The listing builds one solid part. Answer for the finished solid, in the listing's coordinates (mm). Face numbers are marked on the shaded views. Give positions to 0.01 mm unless a question says otherwise; leave off trailing zeros. Order: outer loops, then holes, each group sorted by start corner. A loop starts at its lowest first (then second) coordinate and runs counter-clockwise, first axis right, second up. Notation, with made-up numbers: (20.5, 62) - (62.5, 62) arc R17 ccw to (62.5, 86) - close; hole circle Ø9 at (53, 87). An arc over 180 degrees is marked (long way). Answer as CSV lines item,"result". Start each with the question number.
1. Section A-A on y = -1.5 is taken. Give the vertices of the cut face in (x, z), and give its area (3 significant figures).
2. Section D-D on x = 0 is taken. Give the vertices of the cut face in (y, z) (1 decimal).
3. Section B-B on x = -2.75 is taken. Give the vertices of the cut face in (y, z).
4. Consider line 1 along X through (y, z) = (2.5, 0.2); line 2 along X through (y, z) = (-2.5, 0); line 3 along X through (y, z) = (-3, 0.1). Determine where each line is inside the solid, lowest interval first. Write a range as [from, to].
5. Determine the mould class of the marked faces 1, 2 and 3 for opening direction Y: +Y half, -Y half, draft (parallel to the pull), parting line (faces both ways), or undercut.
from build123d import *

# Parameters (mm, degrees)
BOSS_EXTRUDE1_DEPTH = 0.3175


with BuildPart() as part:
    # Sketch1 → Boss-Extrude1 (new body, symmetric)
    with BuildSketch(Plane.XY):
        with BuildLine():
            Line((-2.31, 0), (-3.124160712, 0))
            ThreePointArc((-3.124160712, 0), (-2.463203432, 1.921720325), (-0.76, 3.030310241))
            Line((-0.76, 3.030310241), (-0.565, 2.239838164))
            ThreePointArc((-0.565, 2.239838164), (0, 2.31), (0.565, 2.239838164))
            Line((0.565, 2.239838164), (0.76, 3.030310241))
            ThreePointArc((0.76, 3.030310241), (2.463203432, 1.921720325), (3.124160712, 0))
            Line((3.124160712, 0), (2.31, 0))
            ThreePointArc((2.31, 0), (2.103247489, -0.955222487), (1.52, -1.739453937))
            Line((1.52, -1.739453937), (1.80501504, -3.733492135))
            ThreePointArc((1.80501504, -3.733492135), (2.089707078, -4.11637794), (2.565878648, -4.086183031))
            ThreePointArc((2.565878648, -4.086183031), (0, 4.825), (-2.565878648, -4.086183031))
            ThreePointArc((-2.565878648, -4.086183031), (-2.089707078, -4.11637794), (-1.80501504, -3.733492135))
            Line((-1.80501504, -3.733492135), (-1.52, -1.739453937))
            ThreePointArc((-1.52, -1.739453937), (-2.103247489, -0.955222487), (-2.31, 0))
        make_face()
    extrude(amount=BOSS_EXTRUDE1_DEPTH, both=True)


solid = part.part
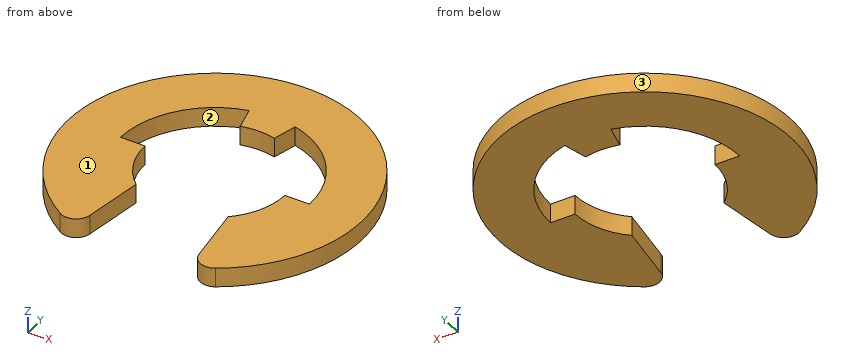
Checks:
1,outline,"(-4.59, -0.32) - (-1.76, -0.32) - (-1.76, 0.32) - (-4.59, 0.32) - close; (1.76, -0.32) - (4.59, -0.32) - (4.59, 0.32) - (1.76, 0.32) - close"
1,area,"3.59 mm²"
2,outline,"(2.3, -0.3) - (4.8, -0.3) - (4.8, 0.3) - (2.3, 0.3) - close"
3,outline,"(-3.96, -0.32) - (0, -0.32) - (0, 0.32) - (-3.96, 0.32) - close; (1.48, -0.32) - (3.96, -0.32) - (3.96, 0.32) - (1.48, 0.32) - close"
4,line 1,"x = [-4.13, -1.87], [-0.63, 0.63], [1.87, 4.13]"
4,line 2,"x = [-4.13, -1.63], [1.63, 4.13]"
4,line 3,"x = [-3.78, -1.7], [1.7, 3.78]"
5,face 1,"draft"
5,face 2,"undercut"
5,face 3,"parting line"
